Design review of the part built by this model. Coordinates are the model's own, in mm. A direction names the side the tool comes from. Give positions to 0.01 mm unless a question says otherwise; leave off trailing zeros. Order: outer loops, then holes, each group sorted by start corner. A loop starts at its lowest first (then second) coordinate and runs counter-clockwise, first axis right, second up. Notation, with made-up numbers: (63, 9) -> (89, 9) arc R30 cw to (89, 42) -> close; hole circle Ø8 at (50.5, 17.5). An arc over 180 degrees is marked (long way). Return JSON: item names as keys, results as strings.
```python
from build123d import *

# Parameters (mm, degrees)
F0_W     = 381
F0_H     = 381
F1_DEPTH = 254
F2_T     = -2.54
F3_W     = 25.4
F3_H     = 25.4
F4_DEPTH = 508


with BuildPart() as f1:
    # F0 (on Top) → F1 (new body)
    with BuildSketch(Plane.XY):
        with Locations((190.5, -190.5)):
            Rectangle(F0_W, F0_H)
    extrude(amount=F1_DEPTH)

    # F2
    f2_openings = [f1.faces().sort_by_distance(p)[0] for p in [
        (190.5, -190.5, 254),
    ]]
    offset(amount=F2_T, openings=f2_openings)

    # F3 (on face) → F4 (join)
    with BuildSketch(Plane(origin=(0, 0, 0), x_dir=(1, 0, 0), z_dir=(0, 0, -1))):
        with Locations((38.1, 342.9)):
            Rectangle(F3_W, F3_H)
        with Locations((342.9, 342.9)):
            Rectangle(F3_W, F3_H)
        with Locations((38.1, 38.1)):
            Rectangle(F3_W, F3_H)
        with Locations((342.9, 38.1)):
            Rectangle(F3_W, F3_H)
    extrude(amount=F4_DEPTH)


solid = f1.part
```
Item 1: Machinability: for faces 1 (the face through (38, -25.4, -250)), 2 (the face through (188, -2.54, 127)), 3 (the face through (38, -50.8, -250)), 4 (the face through (355.6, -38, -250)), 5 (the face through (50.8, -343, -250)), which of the approach directions +Z, -Z, +X, -X, +Y, -Y give a long, thin tool a straight path to every point of the face, cutting with its end or side? Answer none if there is none.
Result set:
{"face 1": "-Z, +X, -X, +Y", "face 2": "+Z", "face 3": "-Z, +X, -X", "face 4": "-Z, +X, +Y, -Y", "face 5": "-Z, +Y, -Y"}
Item 2: Add section C-C (z = 62). Give the boundary of the cut face in (x, y), plus the area to 3 significant figures.
Result set:
{"outline": "(0, -381) -> (381, -381) -> (381, 0) -> (0, 0) -> close; hole (2.54, -378.46) -> (378.46, -378.46) -> (378.46, -2.54) -> (2.54, -2.54) -> close", "area": "3,850 mm^2"}
Item 3: For pin 1 (7.5 mm diameter, centred on x = 349, z = -230, fed in from +Y); pin 2 (12.5 mm diameter, centred on y = -338, z = -272.5, fed in from +X); pin 3 (20.5 mm diameter, centred on x = 337.5, z = -173.5, fed in from -Y), all flat-tipped, find the tip position at first contact; note any pin that passes through.
Result set:
{"pin 1": "stops at y = -25.4", "pin 2": "stops at x = 355.6", "pin 3": "stops at y = -355.6"}
Item 4: Add section D-D (x = 281.5). Give the boundary of the cut face in (y, z), plus the area to 3 significant figures.
Result set:
{"outline": "(-381, 0) -> (0, 0) -> (0, 254) -> (-2.54, 254) -> (-2.54, 2.54) -> (-378.46, 2.54) -> (-378.46, 254) -> (-381, 254) -> close", "area": "2,250 mm^2"}
Item 5: Add section A-A (z = -452). Give the boundary of the cut face in (x, y), plus the area to 3 significant figures.
Result set:
{"outline": "(25.4, -355.6) -> (50.8, -355.6) -> (50.8, -330.2) -> (25.4, -330.2) -> close; (25.4, -50.8) -> (50.8, -50.8) -> (50.8, -25.4) -> (25.4, -25.4) -> close; (330.2, -355.6) -> (355.6, -355.6) -> (355.6, -330.2) -> (330.2, -330.2) -> close; (330.2, -50.8) -> (355.6, -50.8) -> (355.6, -25.4) -> (330.2, -25.4) -> close", "area": "2,580 mm^2"}
Item 6: Mouldability with a two-part tool opening along Y and no side actions: class faces 6 (the face through (343, -330.2, -250)), 7 (the face through (355.6, -343, -250)), 8 (the face through (188, 0, 125)) as released by +Y, released by -Y, zero draft, split by the parting line, or undercut.
Result set:
{"face 6": "undercut", "face 7": "zero draft", "face 8": "released by +Y"}
Item 7: Add section B-B (y = -126). Give the boundary of the cut face in (x, z).
Result set:
{"outline": "(0, 0) -> (381, 0) -> (381, 254) -> (378.46, 254) -> (378.46, 2.54) -> (2.54, 2.54) -> (2.54, 254) -> (0, 254) -> close"}
Item 8: Wall thickness on L1, parallel to Y at x = 269, z = 37; L2, parallel to X at y = -211, z = 14.5; L3, parallel to Y at x = 352.5, z = -82: over which ranges is each line inside the solid? List them lowest first. Write a range as [from, to].
Result set:
{"L1": "y = [-381, -378.46], [-2.54, 0]", "L2": "x = [0, 2.54], [378.46, 381]", "L3": "y = [-355.6, -330.2], [-50.8, -25.4]"}
